```python
from build123d import *

# Parameters (mm, degrees)
SKETCH1_R           = 41.275
BASE_EXTRUDE_DEPTH  = 10.795
SKETCH6_R           = 9.525
BOSS_EXTRUDE2_DEPTH = 156.845
FILLET1_R           = 25.4
CUT_EXTRUDE2_START  = -4.7625
SKETCH9_R           = 3.3734375
CUT_EXTRUDE2_DEPTH  = 162.6075
SKETCH26_R          = 69.037542482
SKETCH26_R_2        = 38.1
CUT_EXTRUDE7_DEPTH  = 1.27
SKETCH19_W          = 6.35
SKETCH19_H          = 9.525
CUT_EXTRUDE6_DEPTH  = 42.275


with BuildPart() as part:
    # Sketch1 → Base-Extrude (new body)
    with BuildSketch(Plane.XY):
        Circle(SKETCH1_R)
    extrude(amount=BASE_EXTRUDE_DEPTH)

    # Sketch6 → Boss-Extrude2 (add)
    with BuildSketch(Plane(origin=(0, 0, 0), x_dir=(-1, 0, 0), z_dir=(0, 0, -1))):
        with Locations(Location((0, 0, 0), (0, 0, 180))):  # turned: the seam where the file's is
            Circle(SKETCH6_R)
    extrude(amount=BOSS_EXTRUDE2_DEPTH)

    # Fillet1
    fillet1_edges = [part.edges().sort_by_distance(p)[0] for p in [
        (-9.525, 0, 0),
    ]]
    fillet(fillet1_edges, radius=FILLET1_R)

    # Sketch9 → Cut-Extrude2 (cut)
    with BuildSketch(Plane(origin=(0, 0, 0), x_dir=(-1, 0, 0), z_dir=(0, 0, -1)).offset(CUT_EXTRUDE2_START)):
        with Locations((34.925, 0)):
            Circle(SKETCH9_R)
    cut_extrude2 = extrude(amount=CUT_EXTRUDE2_DEPTH, mode=Mode.SUBTRACT)

    # Mirror1: Cut-Extrude2 across plane
    add(cut_extrude2.mirror(Plane(origin=(0, 0, 0), x_dir=(0, 0, 1), z_dir=(1, 0, 0))), mode=Mode.SUBTRACT)

    # Sketch26 → Cut-Extrude7 (cut)
    with BuildSketch(Plane.XY.offset(10.795)):
        Circle(SKETCH26_R)
        Circle(SKETCH26_R_2, mode=Mode.SUBTRACT)
    extrude(amount=-CUT_EXTRUDE7_DEPTH, mode=Mode.SUBTRACT)

    # Sketch19 → Cut-Extrude6 (cut, symmetric)
    with BuildSketch(Plane(origin=(0, 0, 0), x_dir=(1, 0, 0), z_dir=(0, 1, 0))):
        with Locations((9.525, 152.0825)):
            Rectangle(SKETCH19_W, SKETCH19_H)
    cut_extrude6 = extrude(amount=CUT_EXTRUDE6_DEPTH, both=True, mode=Mode.SUBTRACT)

    # Mirror2: Cut-Extrude6 across plane
    add(cut_extrude6.mirror(Plane(origin=(0, 0, 0), x_dir=(0, 0, 1), z_dir=(1, 0, 0))), mode=Mode.SUBTRACT)

    # Sketch21 → Cut-Revolve6 (revolve, cut)
    with BuildSketch(Plane(origin=(0, 0, 0), x_dir=(1, 0, 0), z_dir=(0, 1, 0))):
        with BuildLine():
            Line((29.845, -10.795), (0, -10.795))
            Line((0, -10.795), (0, 8.916390985))
            Line((0, 8.916390985), (1.5875, 8.916390985))
            Line((1.5875, 8.916390985), (1.5875, 8.37370061))
            ThreePointArc((1.5875, 8.37370061), (4.306912353, 7.253081359), (6.42537092, 5.212707777))
            ThreePointArc((6.42537092, 5.212707777), (15.158650592, -3.393177249), (26.328076923, -8.450384615))
            ThreePointArc((26.328076923, -8.450384615), (28.287346246, -9.321480631), (29.845, -10.795))
        make_face()
    revolve(axis=Axis((0, 0, 10.795), (0, 0, 1)), mode=Mode.SUBTRACT)

    # Sketch22 → Cut-Revolve7 (revolve, cut)
    with BuildSketch(Plane(origin=(0, 0, 0), x_dir=(1, 0, 0), z_dir=(0, 1, 0))):
        Polygon((8.058530316, 156.845), (9.525, 156.845), (9.525, 154.305), align=None)
    revolve(axis=Axis((0, 0, 10.795), (0, 0, -1)), mode=Mode.SUBTRACT)

    # Sketch23 → Cut-Revolve8 (revolve, cut)
    with BuildSketch(Plane(origin=(0, 0, 0), x_dir=(1, 0, 0), z_dir=(0, 1, 0)), mode=Mode.PRIVATE) as cut_revolve8_sk:
        Polygon((40.259, 0), (41.275, 0), (41.275, -1.016), align=None)
        Polygon((40.259, -9.525), (41.275, -9.525), (41.275, -8.509), align=None)
    revolve(cut_revolve8_sk.sketch.rotate(Axis((0, 0, 10.795), (0, 0, 1)), 180), axis=Axis((0, 0, 10.795), (0, 0, 1)), mode=Mode.SUBTRACT)  # turned: the seam where the file's is


solid = part.part
```
CAD build for the part. Positions are in the model's coordinates, mm. A direction names the side the tool comes from. Round coordinates to 2 decimals unless told otherwise and drop trailing zeros. Write each loop counter-clockwise with the first axis right and the second up, starting at its lowest first coordinate (ties: lowest second). Pieces come first, ordered by that corner, then holes.
Item 1: Drill centre lines: L1, parallel to Z at x = -30.5, y = 8 (3 decimals); L2, parallel to Z at x = -32.5, y = 9 (3 decimals); L3, parallel to Y at x = -3, z = -28.5. Where is each one in solid material? Low to high.
Filled in:
L1: z = -0.228 to 10.795
L2: z = -0.028 to 10.795
L3: y = -9.04 to 9.04
Item 2: Tool access for faces 4 (the flat face through (8, 0, -147.32)), 5 (the cylindrical face through (-30.235, -23.183, 10.169)), 6 (the conical face through (-0.107, 8.455, -156.157)), 7 (the flat face through (-6.35, 0, -152)), 8 (the cylindrical face through (-2.06, 9.3, -88.95)): list every direction of +Z, -Z, +X, -X, +Y, -Y with a clear straight run to the whole face (end or side of a thin tool).
Filled in:
face 4: -Z, +X, +Y, -Y
face 5: +Z
face 6: -Z, +Y
face 7: -Z, -X, +Y, -Y
face 8: -Z
Item 3: Mould opens along X. For faces 1 (the flat face through (6.35, 0, -152)), 2 (the cylindrical face through (-31.555, 0.148, 2.303)), 3 (the flat face through (0, 0, -156.845)) say: released by +X, released by -X, zero draft, split by the parting line, or undercut.
Filled in:
face 1: released by +X
face 2: undercut
face 3: zero draft
Item 4: Band-saw the part on A-A on z = -102.5. Write the cut outline in (x, y) (3 decimals), then the cut area to 3 significant figures.
Filled in:
outline: circle Ø19.05 at (0, 0)
area: 285 mm2
Item 5: Drop flat-ended pins along their axis: pin 1 Ø8 at (x, y) = (-34.925, 0) entering from -Z; pin 2 Ø2.5 at (x, y) = (8.5, 0) entering from -Z; pin 3 Ø7.5 at (x, y) = (-34, 0) entering from -Z. Give the stop position or say it passes through.
Filled in:
pin 1: stops at z = -0.32
pin 2: stops at z = -147.32
pin 3: stops at z = -0.43
